The model under review builds one solid part; all positions refer to its coordinate system, in mm. A direction names the side the tool comes from. Round coordinates to 2 decimals unless told otherwise and drop trailing zeros. Loops run counter-clockwise (first coordinate to the right, second up) from the corner with the lowest first, then second, coordinate; pieces in that order, holes last. Notation, with made-up numbers: M -14,49 L 5,49 A23 ccw 5,63 Z; hole C 1,-10 d3. An arc over 180 degrees is marked long. Answer as a JSON object with one key per item and string values. Group by question number.
Item 1: Consider section C-C (x = -1.5). Give the boundary of the cut face in (y, z).
Item 2: Insertion check: P1, Ø9.5, axis at x = 2.75, y = 2.28, coming from the -Z side; P2, Ø5, axis at y = -3.5, z = 4, coming from the +X side; P3, Ø2, axis at x = -14, y = -3.5, coming from the +Z side. Each pin has a flat end and moves straight along its axis. Give the tip position at first contact, or say it passes through.
Item 3: Tool access review of faces 1 (the face through (27.006, 12.544, 5.288)), 2 (the face through (-2, 8, 0)): name each direction out of +Z, -Z, +X, -X, +Y, -Y from which nothing blocks a thin tool from reaching the whole face with its end or side.
Item 4: The part is to be moulded in two halves that separate along X. For faces 3 (the face through (-23.019, 2, 29)), 4 (the face through (25.037, 2.097, -1.518)), 5 (the face through (-24.005, 7.529, 45.066)), say which applies: +X half, -X half, draft (parallel to the pull), parting line (faces both ways), or undercut.
Item 5: Consider section D-D (x = -11). Give the boundary of the cut face in (y, z), and give its area (3 significant figures).
Item 6: To check wall thickness, follow line 1 (X direction, y = -4, z = 31.5); line 2 (Z direction, x = -1, y = 12.75); line 3 (X direction, y = 7.75, z = 7). State the ranges of each line that lie inside material, in increasing order.
Item 7: Consider section B-B (y = -7.5). Give the boundary of the cut face in (x, z).
Item 8: Consider section A-A (z = 22.5). Give the boundary of the cut face in (x, y).
```python
from build123d import *

# Parameters (mm, degrees)
SKETCH_1_W                       = 42.5
SKETCH_1_H                       = 26
SM_BASE_FLANGE_1_DEPTH           = 2
SM_EDGE_FLANGE_1_STRIP_CUT_DEPTH = 26
SM_EDGE_FLANGE_1_DEPTH           = 26
SM_EDGE_FLANGE_2_STRIP_CUT_DEPTH = 26
SM_EDGE_FLANGE_2_DEPTH           = 26
SM_EDGE_FLANGE_3_STRIP_CUT_DEPTH = 26
SM_EDGE_FLANGE_3_DEPTH           = 26
SM_EDGE_FLANGE_4_STRIP_CUT_DEPTH = 26
SM_EDGE_FLANGE_4_DEPTH           = 26
CUT_EXTRUDE_1_DEPTH              = 100
SKETCH_19_R                      = 1
SKETCH_19_R_2                    = 1.5
SKETCH_19_R_3                    = 4
CUT_EXTRUDE_2_DEPTH              = 100
SKETCH_20_R                      = 6
SKETCH_20_R_2                    = 1.5
CUT_EXTRUDE_3_DEPTH              = 100
SKETCH_21_R                      = 1.5
CUT_EXTRUDE_4_DEPTH              = 2
SKETCH_22_R                      = 1.5
CUT_EXTRUDE_5_DEPTH              = 2
SKETCH_23_R                      = 1.5
CUT_EXTRUDE_6_DEPTH              = 100


# Sheet-metal steps are written as plain solids
with BuildPart() as part:
    # Sketch 1 → 基体-法兰1 (new body)
    with BuildSketch(Plane.XY):
        with Locations((2.752259036, 2.278990964)):
            Rectangle(SKETCH_1_W, SKETCH_1_H)
    extrude(amount=-SM_BASE_FLANGE_1_DEPTH)

    # 边线-法兰1 strip (across the edge) → 边线-法兰1 strip cut (cut)
    with BuildSketch(Plane(origin=(24.002259036, -10.721009036, 0), x_dir=(-0.939692620785907, 0, 0.3420201433256726), z_dir=(0, 1, 0))):
        Polygon((-9.101268459, 1.184235268), (-0.199372324, -2.055789953), (0.484667962, -0.176404712), (-8.417228173, 3.06362051), align=None)
    extrude(amount=SM_EDGE_FLANGE_1_STRIP_CUT_DEPTH, mode=Mode.SUBTRACT)

    # 边线-法兰1 section (across the edge) → 边线-法兰1 (add)
    with BuildSketch(Plane(origin=(24.002259036, -10.721009036, 0), x_dir=(-0.939692620785907, 0, 0.3420201433256726), z_dir=(0, 1, 0))):
        with BuildLine():
            Line((-2, 0.515772873), (-2, 13.219584924))
            Line((-2, 13.219584924), (0, 13.219584924))
            Line((0, 13.219584924), (0, 0.515772873))
            ThreePointArc((0, 0.515772873), (0.133212604, 0.09327647), (0.484667962, -0.176404712))
            Line((0.484667962, -0.176404712), (-0.199372324, -2.055789953))
            ThreePointArc((-0.199372324, -2.055789953), (-1.505091484, -1.053876403), (-2, 0.515772873))
        make_face()
    extrude(amount=SM_EDGE_FLANGE_1_DEPTH)

    # 边线-法兰2 strip (across the edge) → 边线-法兰2 strip cut (cut)
    with BuildSketch(Plane(origin=(28.523623366, -10.721009036, 12.422346403), x_dir=(-1, 0, 0), z_dir=(0, 1, 0))):
        Polygon((-5.074988048, 8.095806265), (-1.834962826, -0.80608987), (0.044422416, -0.122049584), (-3.195602806, 8.779846552), align=None)
    extrude(amount=SM_EDGE_FLANGE_2_STRIP_CUT_DEPTH, mode=Mode.SUBTRACT)

    # 边线-法兰2 section (across the edge) → 边线-法兰2 (add)
    with BuildSketch(Plane(origin=(28.523623366, -10.721009036, 12.422346403), x_dir=(-1, 0, 0), z_dir=(0, 1, 0))):
        with BuildLine():
            Line((-2, 0.129882454), (-2, 41.647346039))
            Line((-2, 41.647346039), (0, 41.647346039))
            Line((0, 41.647346039), (0, 0.129882454))
            ThreePointArc((0, 0.129882454), (0.011190609, 0.001973206), (0.044422416, -0.122049584))
            Line((0.044422416, -0.122049584), (-1.834962826, -0.80608987))
            ThreePointArc((-1.834962826, -0.80608987), (-1.958424897, -0.345323149), (-2, 0.129882454))
        make_face()
    extrude(amount=SM_EDGE_FLANGE_2_DEPTH)

    # 边线-法兰3 strip (across the edge) → 边线-法兰3 strip cut (cut)
    with BuildSketch(Plane(origin=(-18.497740964, 15.278990964, 0), x_dir=(0.939692620785907, 0, 0.3420201433256726), z_dir=(0, -1, 0))):
        Polygon((-9.101268459, 1.184235268), (-0.199372324, -2.055789953), (0.484667962, -0.176404712), (-8.417228173, 3.06362051), align=None)
    extrude(amount=SM_EDGE_FLANGE_3_STRIP_CUT_DEPTH, mode=Mode.SUBTRACT)

    # 边线-法兰3 section (across the edge) → 边线-法兰3 (add)
    with BuildSketch(Plane(origin=(-18.497740964, 15.278990964, 0), x_dir=(0.939692620785907, 0, 0.3420201433256726), z_dir=(0, -1, 0))):
        with BuildLine():
            Line((-2, 0.515772873), (-2, 13.219584924))
            Line((-2, 13.219584924), (0, 13.219584924))
            Line((0, 13.219584924), (0, 0.515772873))
            ThreePointArc((0, 0.515772873), (0.133212604, 0.09327647), (0.484667962, -0.176404712))
            Line((0.484667962, -0.176404712), (-0.199372324, -2.055789953))
            ThreePointArc((-0.199372324, -2.055789953), (-1.505091484, -1.053876403), (-2, 0.515772873))
        make_face()
    extrude(amount=SM_EDGE_FLANGE_3_DEPTH)

    # 边线-法兰4 strip (across the edge) → 边线-法兰4 strip cut (cut)
    with BuildSketch(Plane(origin=(-23.019105294, 15.278990964, 12.422346403), x_dir=(1, 0, 0), z_dir=(0, -1, 0))):
        Polygon((-5.074988048, 8.095806265), (-1.834962826, -0.80608987), (0.044422416, -0.122049584), (-3.195602806, 8.779846552), align=None)
    extrude(amount=SM_EDGE_FLANGE_4_STRIP_CUT_DEPTH, mode=Mode.SUBTRACT)

    # 边线-法兰4 section (across the edge) → 边线-法兰4 (add)
    with BuildSketch(Plane(origin=(-23.019105294, 15.278990964, 12.422346403), x_dir=(1, 0, 0), z_dir=(0, -1, 0))):
        with BuildLine():
            Line((-2, 0.129882454), (-2, 41.647346039))
            Line((-2, 41.647346039), (0, 41.647346039))
            Line((0, 41.647346039), (0, 0.129882454))
            ThreePointArc((0, 0.129882454), (0.011190609, 0.001973206), (0.044422416, -0.122049584))
            Line((0.044422416, -0.122049584), (-1.834962826, -0.80608987))
            ThreePointArc((-1.834962826, -0.80608987), (-1.958424897, -0.345323149), (-2, 0.129882454))
        make_face()
    extrude(amount=SM_EDGE_FLANGE_4_DEPTH)

    # 草图18 → 切除-拉伸1 (cut)
    with BuildSketch(Plane(origin=(30.523623366, 0, 0), x_dir=(0, 0, -1), z_dir=(1, 0, 0))):
        with BuildLine():
            Line((-41.069692441, 15.278990964), (-54.069692441, 15.278990964))
            Line((-54.069692441, 15.278990964), (-54.069692441, 2.278990964))
            ThreePointArc((-54.069692441, 2.278990964), (-50.262080597, 11.471379119), (-41.069692441, 15.278990964))
        make_face()
        with BuildLine():
            ThreePointArc((-41.069692441, -10.721009036), (-50.262080597, -6.913397192), (-54.069692441, 2.278990964))
            Line((-54.069692441, 2.278990964), (-54.069692441, -10.721009036))
            Line((-54.069692441, -10.721009036), (-41.069692441, -10.721009036))
        make_face()
    extrude(amount=-CUT_EXTRUDE_1_DEPTH, mode=Mode.SUBTRACT)

    # 草图19 → 切除-拉伸2 (cut)
    with BuildSketch(Plane(origin=(30.523623366, 0, 0), x_dir=(0, 0, -1), z_dir=(1, 0, 0))):
        with Locations((-36.119944973, 7.228738432)):
            Circle(SKETCH_19_R)
        with Locations((-34.069692441, 2.278990964)):
            Circle(SKETCH_19_R_2)
        with Locations((-36.119944973, -2.670756504)):
            Circle(SKETCH_19_R)
        with Locations((-41.069692441, -4.721009036)):
            Circle(SKETCH_19_R_2)
        with Locations((-46.019439909, -2.670756504)):
            Circle(SKETCH_19_R)
        with Locations((-48.069692441, 2.278990964)):
            Circle(SKETCH_19_R_2)
        with Locations((-46.019439909, 7.228738432)):
            Circle(SKETCH_19_R)
        with Locations((-41.069692441, 9.278990964)):
            Circle(SKETCH_19_R_2)
        with Locations((-41.069692441, 2.278990964)):
            Circle(SKETCH_19_R_3)
    extrude(amount=-CUT_EXTRUDE_2_DEPTH, mode=Mode.SUBTRACT)

    # 草图20 → 切除-拉伸3 (cut)
    with BuildSketch(Plane.XY):
        with Locations((2.752259036, 2.278990964)):
            Circle(SKETCH_20_R)
        with Locations((9.469773457, 8.996505385)):
            Circle(SKETCH_20_R_2)
        with Locations((-3.965255385, 8.996505385)):
            Circle(SKETCH_20_R_2)
        with Locations((-3.965255385, -4.438523457)):
            Circle(SKETCH_20_R_2)
        with Locations((9.469773457, -4.438523457)):
            Circle(SKETCH_20_R_2)
    extrude(amount=-CUT_EXTRUDE_3_DEPTH, mode=Mode.SUBTRACT)

    # 草图21 → 切除-拉伸4 (cut)
    with BuildSketch(Plane(origin=(23.073913338, 0, -8.398217643), x_dir=(-0.3420201433256726, 0, -0.9396926207859071), z_dir=(0.9396926207859071, 0, -0.3420201433256726))):
        with Locations((-15.011993747, 11.278990964)):
            Circle(SKETCH_21_R)
        with Locations((-15.011993747, -6.721009036)):
            Circle(SKETCH_21_R)
    extrude(amount=-CUT_EXTRUDE_4_DEPTH, mode=Mode.SUBTRACT)

    # 草图22 → 切除-拉伸5 (cut)
    with BuildSketch(Plane(origin=(-18.213301561, 0, -6.629099636), x_dir=(-0.3420201433256726, 0, 0.9396926207859071), z_dir=(-0.9396926207859071, 0, -0.3420201433256726))):
        with Locations((13.129337687, 11.278990964)):
            Circle(SKETCH_22_R)
        with Locations((13.129337687, -6.721009036)):
            Circle(SKETCH_22_R)
    extrude(amount=-CUT_EXTRUDE_5_DEPTH, mode=Mode.SUBTRACT)

    # 草图23 → 切除-拉伸6 (cut)
    with BuildSketch(Plane.ZY.offset(25.019105294)):
        with Locations((18.552228857, 2.278990964)):
            Circle(SKETCH_23_R)
    extrude(amount=-CUT_EXTRUDE_6_DEPTH, mode=Mode.SUBTRACT)


solid = part.part
```
Geometry results:
{
 "1": {"outline": "M -10.72,-2 L -1.95,-2 L -1.95,0 L -10.72,0 Z; M 6.51,-2 L 15.28,-2 L 15.28,0 L 6.51,0 Z"},
 "2": {"P1": "passes through", "P2": "stops at x = 28.5", "P3": "stops at z = 0"},
 "3": {"face 1": "none", "face 2": "+Z, +Y, -Y"},
 "4": {"face 3": "undercut", "face 4": "+X half", "face 5": "draft"},
 "5": {"outline": "M -10.72,-2 L 15.28,-2 L 15.28,0 L -10.72,0 Z", "area": "52.0 mm^2"},
 "6": {"line 1": "x = -25.02 to -23.02, 28.52 to 30.52", "line 2": "z = -2 to 0", "line 3": "x = -23.17 to -21.05, 26.55 to 28.68"},
 "7": {"outline": "M -25.02,12.55 A2.74 ccw -24.85,11.62 L -23.14,6.91 L -21.26,7.6 L -22.97,12.3 A0.74 cw -23.02,12.55 L -23.02,49.64 L -25.02,49.64 Z; M -22.27,4.5 L -20.55,-0.2 A2.74 ccw -17.98,-2 L 23.49,-2 A2.74 ccw 26.06,-0.2 L 27.77,4.5 L 25.89,5.19 L 24.18,0.48 A0.74 cw 23.49,0 L -17.98,0 A0.74 cw -18.67,0.48 L -20.39,5.19 Z; M 26.77,7.6 L 28.65,6.91 L 30.36,11.62 A2.74 ccw 30.52,12.55 L 30.52,49.64 L 28.52,49.64 L 28.52,12.55 A0.74 cw 28.48,12.3 Z"},
 "8": {"outline": "M -25.02,-10.72 L -23.02,-10.72 L -23.02,15.28 L -25.02,15.28 Z; M 28.52,-10.72 L 30.52,-10.72 L 30.52,15.28 L 28.52,15.28 Z"}
}
